Read the model definition and answer for the solid it produces. Units are mm, in the model's axes. Face numbers are marked on the shaded views. A direction names the side the tool comes from. Coordinates: 2 decimals unless noted, no trailing zeros. Loops run counter-clockwise (first coordinate to the right, second up) from the corner with the lowest first, then second, coordinate; pieces in that order, holes last.
Q1. Straight lines are drawn through the part: line 1 (X direction, y = 3.2, z = 0); line 2 (X direction, y = 2, z = 1.5); line 3 (Z direction, x = 15, y = 3.4). For each, find the intervals that lie inside material, in ascending order.
Q2. Which of the six approach directions +Z, -Z, +X, -X, +Y, -Y give full straight-line access (tool end or side, diameter ignored) to the marked faces 5 and 6?
Q3. Flat-ended cylindrical pins translate along their axes: P1, Ø0.6, axis at x = 7.5, z = 5, coming from the +Y side; P2, Ø0.8, axis at x = 5.5, z = 7, coming from the -Y side; P3, Ø3, axis at x = -15, z = 0, coming from the -Y side. Find the tip coordinate at first contact, or state that the pin passes through.
Q4. Section C-C (y = 1.5) is taken. Count the separate pieces of the cut face and the enclosed holes in it, then the cut area to 3 significant figures.
Q5. Section A-A (z = 0) is taken. Give the vertices of the cut face in (x, y).
Q6. The mould has two halves that part along Z. Classify the marked faces 1, 2, 3 and 4: pulls with the +Z half, pulls with the -Z half, needs draft (parallel to the pull), parting line crosses it, or undercut.
Q7. Section B-B (x = 3) is taken. Give the vertices of the cut face in (y, z).
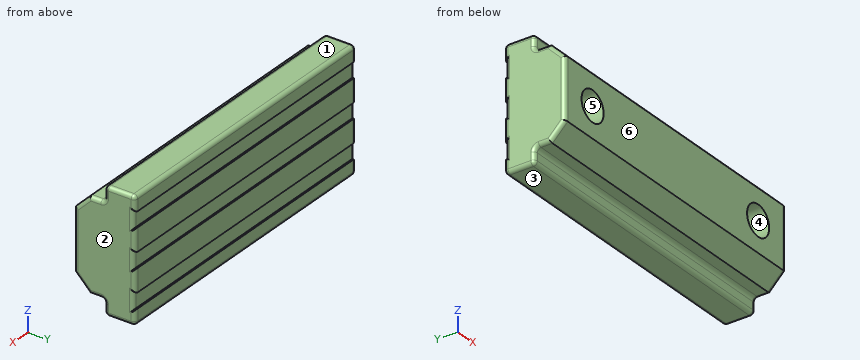
from build123d import *

# Parameters (mm, degrees)
ESQUISSE1_W             = 40
ESQUISSE1_H             = 8
BOSS_EXTRU_1_DEPTH      = 8
BOSS_EXTRU_3_DEPTH      = 40
ESQUISSE6_W             = 40
ESQUISSE6_H             = 4
BOSS_EXTRU_4_DEPTH      = 2
ESQUISSE7_R             = 2
ENL_V_MAT_EXTRU_1_DEPTH = 6
ESQUISSE10_W            = 40
ESQUISSE10_H            = 2
ENL_V_MAT_EXTRU_4_DEPTH = 0.2
CONG_2_R                = 0.5
CONG_3_R                = 0.5
CONG_4_R                = 0.5


with BuildPart() as part:
    # Esquisse1 → Boss.-Extru.1 (new body)
    with BuildSketch(Plane(origin=(0, 0, 0), x_dir=(1, 0, 0), z_dir=(0, 1, 0))):
        Rectangle(ESQUISSE1_W, ESQUISSE1_H)
    extrude(amount=BOSS_EXTRU_1_DEPTH)

    # Esquisse5 → Boss.-Extru.3 (add)
    with BuildSketch(Plane.ZY.offset(20)):
        Polygon((-4, 0), (-6, 2), (-6, 8), (-4, 8), align=None)
    boss_extru_3 = extrude(amount=-BOSS_EXTRU_3_DEPTH)

    # Symétrie2: Boss.-Extru.3 across plane
    add(boss_extru_3.mirror(Plane(origin=(0, 0, 0), x_dir=(1, 0, 0), z_dir=(0, 0, -1))))

    # Esquisse6 → Boss.-Extru.4 (add)
    with BuildSketch(Plane(origin=(0, 0, -6), x_dir=(-1, 0, 0), z_dir=(0, 0, -1))):
        with Locations((0, 6)):
            Rectangle(ESQUISSE6_W, ESQUISSE6_H)
    boss_extru_4 = extrude(amount=BOSS_EXTRU_4_DEPTH)

    # Symétrie4: Boss.-Extru.4 across plane
    add(boss_extru_4.mirror(Plane(origin=(0, 0, 0), x_dir=(1, 0, 0), z_dir=(0, 0, -1))))

    # Esquisse7 → Enlèv. mat.-Extru.1 (cut)
    with BuildSketch(Plane.XZ):
        with Locations(Location((-15, 0, 0), (0, 0, 270))):
            Circle(ESQUISSE7_R)
    enl_v_mat_extru_1 = extrude(amount=-ENL_V_MAT_EXTRU_1_DEPTH, mode=Mode.SUBTRACT)

    # Symétrie10: Enlèv. mat.-Extru.1 across plane
    add(enl_v_mat_extru_1.mirror(Plane(origin=(0, 0, 0), x_dir=(0, 0, 1), z_dir=(1, 0, 0))), mode=Mode.SUBTRACT)

    # Esquisse10 → Enlèv. mat.-Extru.4 (cut)
    with BuildSketch(Plane(origin=(0, 8, 0), x_dir=(1, 0, 0), z_dir=(0, 1, 0))):
        Rectangle(ESQUISSE10_W, ESQUISSE10_H)
        with Locations((0, 5)):
            Rectangle(ESQUISSE10_W, ESQUISSE10_H)
        with Locations((0, -5)):
            Rectangle(ESQUISSE10_W, ESQUISSE10_H)
    extrude(amount=-ENL_V_MAT_EXTRU_4_DEPTH, mode=Mode.SUBTRACT)

    # Congé2
    cong_2_edges = [part.edges().sort_by_distance(p)[0] for p in [
        (0, 8, -8),
        (0, 8, 8),
    ]]
    fillet(cong_2_edges, radius=CONG_2_R)

    # Congé3
    cong_3_edges = [part.edges().sort_by_distance(p)[0] for p in [
        (0, 4, -6),
        (0, 4, -8),
        (0, 4, 8),
        (0, 4, 6),
    ]]
    fillet(cong_3_edges, radius=CONG_3_R)

    # Congé4
    cong_4_edges = [part.edges().sort_by_distance(p)[0] for p in [
        (-20, 7.8, -5),
        (-20, 7.9, -4),
        (-20, 7.9, -6),
        (20, 7.8, -5),
        (20, 7.9, -6),
        (20, 7.9, -4),
        (-20, 7.8, 5),
        (-20, 7.9, 6),
        (-20, 7.9, 4),
        (20, 7.8, 5),
        (20, 7.9, 4),
        (20, 7.9, 6),
        (20, 8, 6.75),
        (20, 6, 8),
        (20, 6, -8),
        (20, 7.853553391, -7.853553391),
        (20, 7.853553391, 7.853553391),
        (-20, 8, -6.75),
        (-20, 7.853553391, -7.853553391),
        (-20, 7.853553391, 7.853553391),
        (20, 2.75, 6),
        (-20, 2.75, 6),
        (20, 4, 7),
        (-20, 4, 7),
        (20, 1, -5),
        (-20, 6, 8),
        (-20, 6, -8),
        (-20, 4, -7),
        (-20, 2.75, -6),
        (-20, 4.146446609, -7.853553391),
        (-20, 4.146446609, 7.853553391),
        (20, 2.75, -6),
        (20, 4, -7),
        (20, 4.146446609, -7.853553391),
        (20, 4.146446609, 7.853553391),
        (-20, 3.853553391, 6.146446609),
        (20, 3.853553391, 6.146446609),
        (-20, 3.853553391, -6.146446609),
        (20, 3.853553391, -6.146446609),
        (-20, 1, -5),
        (-20, 1, 5),
        (20, 1, 5),
        (-20, 0, 0),
        (20, 0, 0),
        (20, 8, -2.5),
        (-20, 8, 2.5),
        (-20, 7.8, 0),
        (-20, 7.9, 1),
        (-20, 7.9, -1),
        (20, 7.8, 0),
        (20, 7.9, -1),
        (20, 7.9, 1),
        (-20, 8, 6.75),
        (20, 8, 2.5),
        (-20, 8, -2.5),
        (20, 8, -6.75),
    ]]
    fillet(cong_4_edges, radius=CONG_4_R)


solid = part.part
Numbers:
1. line 1: x = -20 to -17, -13 to 13, 17 to 20
1. line 2: x = -20 to -16.32, -13.68 to 13.68, 16.32 to 20
1. line 3: z = -6 to -2, 2 to 6
2. face 5: -Y
2. face 6: +Z, -Z, +X, -X, -Y
3. P1: stops at y = 7.8
3. P2: stops at y = 4
3. P3: stops at y = 6
4. separate pieces: 1
4. enclosed holes: 2
4. area: 415 mm2
5. outline: (-20, 0.5) arc R0.5 ccw to (-19.5, 0) - (-17, 0) - (-17, 6) - (-13, 6) - (-13, 0) - (13, 0) - (13, 6) - (17, 6) - (17, 0) - (19.5, 0) arc R0.5 ccw to (20, 0.5) - (20, 7.3) arc R0.5 ccw to (19.5, 7.8) - (-19.5, 7.8) arc R0.5 ccw to (-20, 7.3) - close
6. face 1: pulls with the +Z half
6. face 2: needs draft
6. face 3: pulls with the -Z half
6. face 4: undercut
7. outline: (0, -4) - (2, -6) - (3.5, -6) arc R0.5 cw to (4, -6.5) - (4, -7.5) arc R0.5 ccw to (4.5, -8) - (7.5, -8) arc R0.5 ccw to (8, -7.5) - (8, -6) - (7.8, -6) - (7.8, -4) - (8, -4) - (8, -1) - (7.8, -1) - (7.8, 1) - (8, 1) - (8, 4) - (7.8, 4) - (7.8, 6) - (8, 6) - (8, 7.5) arc R0.5 ccw to (7.5, 8) - (4.5, 8) arc R0.5 ccw to (4, 7.5) - (4, 6.5) arc R0.5 cw to (3.5, 6) - (2, 6) - (0, 4) - close
